from build123d import *

# Parameters (mm, degrees)
F0_W           = 150
F0_H           = 75
F1_DEPTH       = 400
F2_R           = 15
F4_D           = 5.5
F4_DEPTH       = 12
F4_CSINK_D     = 11.2
F4_CSINK_ANGLE = 90
F4_TIP         = 1.6523667023
F5_R           = 10


with BuildPart() as f1:
    # F0 (on Front) → F1 (new body)
    with BuildSketch(Plane.XZ):
        Rectangle(F0_W, F0_H)
    extrude(amount=F1_DEPTH)

    # F2
    f2_edges = [f1.edges().sort_by_distance(p)[0] for p in [
        (75, -200, 37.5),
        (75, -200, -37.5),
        (-75, -200, 37.5),
        (-75, -200, -37.5),
    ]]
    fillet(f2_edges, radius=F2_R)

    # F4
    with Locations(Plane.XZ.offset(400)):
        with Locations((0, 0)):
            CounterSinkHole(F4_D / 2, F4_CSINK_D / 2, depth=F4_DEPTH, counter_sink_angle=F4_CSINK_ANGLE)
            with Locations((0, 0, -(F4_DEPTH + F4_TIP / 2))):  # 118° drill point
                Cone(0, F4_D / 2, F4_TIP, mode=Mode.SUBTRACT)

    # F5
    f5_edges = [f1.edges().sort_by_distance(p)[0] for p in [
        (0, -400, 37.5),
    ]]
    fillet(f5_edges, radius=F5_R)


solid = f1.part
Part model, mm, in its own coordinate system. Give positions to 0.01 mm unless a question says otherwise; leave off trailing zeros. Loops run counter-clockwise (first coordinate to the right, second up) from the corner with the lowest first, then second, coordinate; pieces in that order, holes last. Notation, with made-up numbers: (-21, -18.5) -> (10, -18.5) arc R19 cw to (10, -7.5) -> close; hole circle Ø10 at (-3.5, 74.25). An arc over 180 degrees is marked (long way). Write each question's results on one line, items separated by ' | '. Start each with the question number.
Q1. Pin check, flat tip, straight feed: P1, Ø8, axis at x = 7.5, z = -18.5, coming from the +Y side. Stop position of the tip, or through.
Q2. Wall check: L1, parallel to X at y = -391.25, z = 0; L2, parallel to X at y = -390.25, z = 0; L3, parallel to Z at x = 0, y = -394. Give the ranges that are in metal, low to high.
Q3. Pull direction Z, two halves, no side cores. Call faces 1 (the face through (-1, -192, -37.5)), 2 (the face through (-70.72, -197.73, 32.99)), 3 (the face through (-2.755, -397.288, 0.868)): +Z half, -Z half, draft (parallel to the pull), parting line (faces both ways), or undercut.
Q4. Band-saw the part on A-A on y = -351. List the corners of the cut face in (x, z).
Results are:
1) P1: stops at y = 0
2) L1: x = -74.92 to -2.75, 2.75 to 74.92 | L2: x = -75 to -2.75, 2.75 to 75 | L3: z = -36.67 to -2.75, 2.75 to 36.67
3) face 1: -Z half | face 2: +Z half | face 3: undercut
4) outline: (-75, -22.5) arc R15 ccw to (-60, -37.5) -> (60, -37.5) arc R15 ccw to (75, -22.5) -> (75, 22.5) arc R15 ccw to (60, 37.5) -> (-60, 37.5) arc R15 ccw to (-75, 22.5) -> close
